Here's how the part is built. I have some questions about the finished solid (model axes, mm). Face numbers are marked on the shaded views. A direction names the side the tool comes from. Give positions to 0.01 mm unless a question says otherwise; leave off trailing zeros. Order: outer loops, then holes, each group sorted by start corner. A loop starts at its lowest first (then second) coordinate and runs counter-clockwise, first axis right, second up.
Autodesk Fusion 360 part; units mm, degrees
sketch "Sketch1" plane through (0, 0, 0) normal (0, 1, 0) x (1, 0, 0)
  line L0 (-20, 0) -> (20, 0)
  line L1 (20, 0) -> (20, -5)
  line L2 (20, -5) -> (-20, -5)
  line L3 (-20, -5) -> (-20, 0)
  circle A0 centre (0, -5) radius 5
  circle A1 centre (0, -5) radius 3.6
  circle A2 centre (0, -5) radius 2.2
  dimension "d19" = 10
  dimension "d20" = 7.2
  dimension "d21" = 4.4
extrude "Extrude13" add sketch "Sketch1" along normal blind 20 contours L0 L2 L3 A0
extrude "Extrude14" add sketch "Sketch1" along normal blind 15 contours L2 A0 A1 | L2 A0 A1 | L2 A1 A2 | L2 A1 A2
sketch "Sketch8" plane through (0, 0, 0) normal (0, -1, 0) x (1, 0, 0)
  circle A0 centre (0, 5) radius 2.2
  line L0 (-20, 0) -> (0, 0)
  arc A1 (0, 0) -> (-5, 5) centre (0, 5) ccw
  line L1 (-5, 5) -> (-20, 5)
  circle A2 centre (0, 5) radius 5
  line L2 (-20, 5) -> (-20, 0)
extrude "Extrude15" cut sketch "Sketch8" against normal blind 5 contours A1 A2
extrude "Extrude21" cut 1 faces at (0.2994, 15, 0.9534) along direction (0, -1, 0) blind 1
extrude "Extrude22" cut 1 faces at (0.2994, 5, 0.9534) along direction (0, 1, 0) blind 1
sketch "Sketch12" plane through (0, 0, 5) normal (0, 0, 1) x (-1, 0, 0)
  line L0 (20, 0) -> (5, 0)
  line L1 (5, 0) -> (5, -6)
  line L2 (5, -6) -> (5, -14)
  line L3 (5, -14) -> (5, -20)
  line L4 (5, -20) -> (20, -20)
  line L5 (20, -20) -> (20, 0)
  circle A0 centre (20, -10) radius 10
  circle A1 centre (20, -10) radius 3.6
  circle A2 centre (20, -10) radius 2.2
  dimension "d92" = 20
  dimension "d95" = 7.2
  dimension "d96" = 4.4
extrude "Extrude24" add sketch "Sketch12" against normal blind 5 contours L5 A0 A1 | L5 A1 A2 | L5 A2 picked at (27.8205, -10.6452) picked at (23.1211, -10.1708) picked at (20.6671, -9.6954)
extrude "Extrude25" cut sketch "Sketch12" against normal blind 4.2 contours L5 A1 A2 | L5 A1 A2
extrude "Extrude26" cut sketch "Sketch12" against normal through all contours L5 A2 | L5 A2
fillet "Fillet13" radius 2 1 edges at (-5, 10, 5)
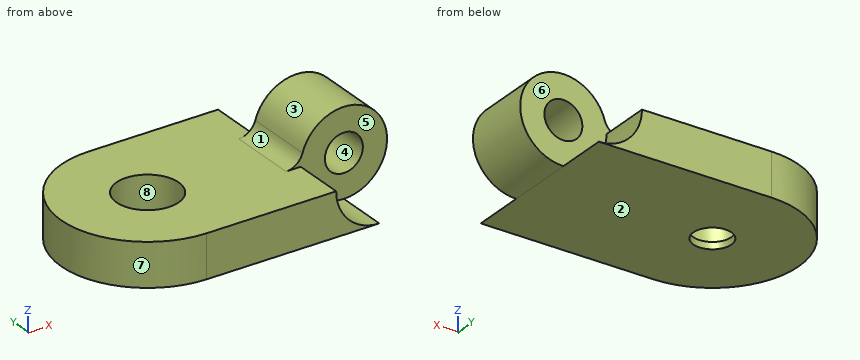
Q1. Thinking about a two-plate mould opening in X: for the marked faces 1, 2, 3 and 4, which applies, released by +X, released by -X, zero draft, split by the parting line, or undercut?
Filled sheet:
face 1: released by -X
face 2: zero draft
face 3: split by the parting line
face 4: undercut
Q2. I need wall thicknesses on L1, parallel to Z at x = 0, y = 10.75; L2, parallel to Y at x = -20, z = 3.25; L3, parallel to Z at x = -12.5, y = 4.5. Which ranges of each line are inside material? Lowest first, please.
Filled sheet:
L1: z = 0 to 2.8, 7.2 to 10
L2: y = 0 to 6.4, 13.6 to 20
L3: z = 0 to 5
Q3. If we section it at A-A on y = 10: List the corners of the cut face in (x, z) for me, plus the area to 3 significant figures.
Filled sheet:
outline: (-30, 0) - (-22.2, 0) - (-22.2, 0.8) - (-23.6, 0.8) - (-23.6, 5) - (-30, 5) - close; (-17.8, 0) - (0, 0) arc R5 ccw (long way) to (-4.79, 6.43) arc R2 cw to (-6.71, 5) - (-16.4, 5) - (-16.4, 0.8) - (-17.8, 0.8) - close; hole circle Ø4.4 at (0, 5)
area: 160 mm2
Q4. If we section it at C-C on x = -13.5: List the corners of the cut face in (y, z) for me.
Filled sheet:
outline: (0, 0) - (20, 0) - (20, 5) - (0, 5) - close
Q5. If we section it at D-D on y = 17.25: List the corners of the cut face in (x, z) for me.
Filled sheet:
outline: (-26.89, 0) - (0, 0) arc R5 cw to (-5, 5) - (-26.89, 5) - close
Q6. If we section it at B-B on z = 3.75: List the corners of the cut face in (x, y) for me.
Filled sheet:
outline: (-20, 0) - (-4.84, 0) - (-4.84, 6) - (-1.81, 6) - (-1.81, 14) - (-4.84, 14) - (-4.84, 20) - (-20, 20) arc R10 ccw to start; (1.81, 6) - (4.84, 6) - (4.84, 14) - (1.81, 14) - close; hole circle Ø7.2 at (-20, 10)
Q7. For the marked faces 5, 6, 7 and 8, which set-ups out of +Z, -Z, +X, -X, +Y, -Y let a thin tool reach every point of the face, with its end or its side?
Filled sheet:
face 5: +Z, +X, -Y
face 6: +Z, +X, +Y
face 7: +Z, -Z, -X
face 8: +Z
Q8. I'm going to push flat-ended pins straight in: P1, Ø6.5, axis at x = -20, y = 10, coming from the +Z side; P2, Ø1.5, axis at x = -2.5, z = 7.5, coming from the -Y side; P3, Ø1, axis at x = -26.5, z = 2, coming from the +Y side. Where does each tip first touch, or does it pass through?
Filled sheet:
P1: stops at z = 0.8
P2: stops at y = 6
P3: stops at y = 18
